Geometry check sheet. Reference: the model listing, model coordinates, mm. Face numbers are marked on the shaded views. A direction names the side the tool comes from. Round coordinates to 2 decimals unless told otherwise and drop trailing zeros. Write each loop counter-clockwise with the first axis right and the second up, starting at its lowest first coordinate (ties: lowest second). Pieces come first, ordered by that corner, then holes. Notation, with made-up numbers: (11, -39.5) -> (32, -39.5) arc R21 ccw to (32, -14.5) -> close; hole circle Ø1 at (58.5, 67.25). An arc over 180 degrees is marked (long way). Use a Markdown table: item, result.
```python
from build123d import *

# Parameters (mm, degrees)
F0_R     = 7.9375
F1_DEPTH = 96.012
F2_DEPTH = 31.75
F3_W     = 25.4
F3_H     = 19.304
F3_W_2   = 28.956
F3_H_2   = 13.716
F4_DEPTH = 51.562
F6_DEPTH = 69.088


with BuildPart() as f1:
    # F0 (on Right) → F1 (new body)
    with BuildSketch(Plane.YZ):
        Polygon((0, 6.604), (0, 0), (56.896, 0), (56.896, 50.8), (44.196, 50.8), align=None)
        with Locations((37.592, 15.748)):
            Circle(F0_R, mode=Mode.SUBTRACT)
        with Locations((37.592, 15.748)):
            Circle(F0_R)
    extrude(amount=-F1_DEPTH)

    # F0 (on Right) → F2 (cut)
    with BuildSketch(Plane.YZ):
        with Locations((37.592, 15.748)):
            Circle(F0_R)
    extrude(amount=-F2_DEPTH, mode=Mode.SUBTRACT)

    # F3 (on face) → F4 (cut)
    with BuildSketch(Plane(origin=(0, 0, 0), x_dir=(1, 0, 0), z_dir=(0, 0, -1))):
        with Locations((-12.7, -9.652)):
            Rectangle(F3_W, F3_H)
        with Locations((-56.134, -6.858)):
            Rectangle(F3_W_2, F3_H_2)
    extrude(amount=-F4_DEPTH, mode=Mode.SUBTRACT)

    # F5 (on face) → F6 (cut)
    with BuildSketch(Plane(origin=(0, 56.896, 0), x_dir=(-1, 0, 0), z_dir=(0, 1, 0))):
        Polygon((18.796, 50.8), (0, 50.8), (0, 32.004), align=None)
        Polygon((96.012, 50.8), (47.244, 50.8), (79.799627, 32.004), (96.012, 32.004), align=None)
    extrude(amount=-F6_DEPTH, mode=Mode.SUBTRACT)


solid = f1.part
```
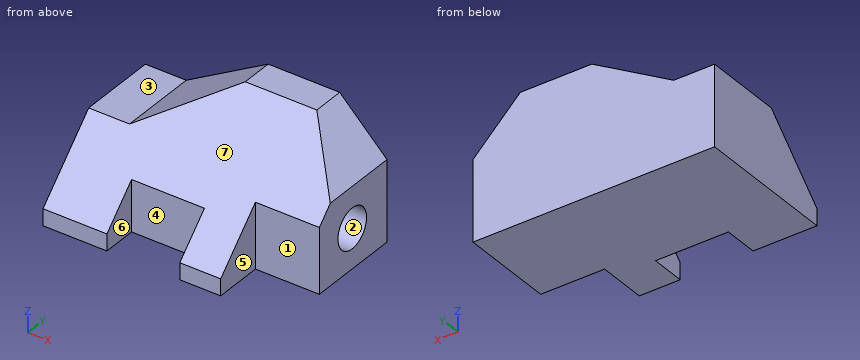
(1) Release check for a two-part mould opening along X. For the marked faces 5, 6 and 7 record: +X half, -X half, draft (parallel to the pull), parting line (faces both ways), or undercut.
A:
| item | result |
|---|---|
| face 5 | +X half |
| face 6 | undercut |
| face 7 | draft |
(2) Gauge pin test, flat ends, axial feed: pin 1 Ø6 at (x, y) = (-29.5, 40) entering from +Z; pin 2 Ø6 at (x, y) = (-81, 43.5) entering from +Z; pin 3 Ø8 at (y, z) = (36.5, 17) entering from +X. Record the tip position at first contact, or that the pin passes through.
A:
| item | result |
|---|---|
| pin 1 | stops at z = 49.6 |
| pin 2 | stops at z = 33.04 |
| pin 3 | stops at x = -31.75 |
(3) Section check A-A on y = 47.5. Record the cut outline in (x, z).
A:
| item | result |
|---|---|
| outline | (-96.01, 0) -> (0, 0) -> (0, 32) -> (-18.8, 50.8) -> (-47.24, 50.8) -> (-79.8, 32) -> (-96.01, 32) -> close |
(4) Section check C-C on x = -35. Record the cut outline in (y, z).
A:
| item | result |
|---|---|
| outline | (0, 0) -> (56.9, 0) -> (56.9, 50.8) -> (44.2, 50.8) -> (0, 6.6) -> close |
(5) Section check D-D on x = -20. Record the cut outline in (y, z) (1 decimal), plus the area to 3 significant figures.
A:
| item | result |
|---|---|
| outline | (19.3, 0) -> (56.9, 0) -> (56.9, 50.8) -> (44.2, 50.8) -> (19.3, 25.9) -> close; hole circle Ø15.9 at (37.6, 15.7) |
| area | 1,400 mm2 |
(6) Access from +Z, -Z, +X, -X, +Y, -Y to the whole of each face (thin tool, end or side, straight path). Record for the marked faces 1, 2, 3 and 4.
A:
| item | result |
|---|---|
| face 1 | +Z, -Z, +X, -Y |
| face 2 | +X |
| face 3 | +Z, -X, +Y, -Y |
| face 4 | +Z, -Z, -Y |
(7) Section check B-B on y = 5. Record the cut outline in (x, z), plus the area to 3 significant figures.
A:
| item | result |
|---|---|
| outline | (-96.01, 0) -> (-70.61, 0) -> (-70.61, 11.6) -> (-96.01, 11.6) -> close; (-41.66, 0) -> (-25.4, 0) -> (-25.4, 11.6) -> (-41.66, 11.6) -> close |
| area | 483 mm2 |
(8) Thickness scan on line 1 (X direction, y = 6, z = 7); line 2 (Y direction, x = -16.5, z = 6); line 3 (Z direction, x = -13.5, y = 46.5). Record the ranges inside material, lowest first.
A:
| item | result |
|---|---|
| line 1 | x = -96.01 to -70.61, -41.66 to -25.4 |
| line 2 | y = 19.3 to 56.9 |
| line 3 | z = 0 to 45.5 |
